from build123d import *
from build123d.topology import SkipClean

# Parameters (mm, degrees)
SKETCH1_R           = 6
BOSS_EXTRUDE1_DEPTH = 5
BOSS_EXTRUDE2_START = -5
BOSS_EXTRUDE2_DEPTH = 5
CUT_EXTRUDE1_START  = -3
SKETCH3_R           = 4.075
CUT_EXTRUDE1_DEPTH  = 3
SKETCH4_W           = 12
SKETCH4_H           = 5
BOSS_EXTRUDE3_DEPTH = 26.5
FILLET1_R           = 6
CUT_EXTRUDE2_DEPTH  = 0.5


with BuildPart() as part:
    # Sketch1 → Boss-Extrude1 (new body)
    with BuildSketch(Plane.XY):
        Circle(SKETCH1_R)
        with BuildLine():
            Line((-2.837252192, 2.925), (2.837252192, 2.925))
            ThreePointArc((2.837252192, 2.925), (0, -4.075), (-2.837252192, 2.925))
        make_face(mode=Mode.SUBTRACT)
    extrude(amount=BOSS_EXTRUDE1_DEPTH)

    # Sketch2 → Boss-Extrude2 (add)
    with BuildSketch(Plane.XY.offset(5).offset(BOSS_EXTRUDE2_START)):
        with BuildLine():
            Line((-6, 0), (-6, 45.2))
            Line((-6, 45.2), (6, 45.2))
            Line((6, 45.2), (6, 0))
            ThreePointArc((6, 0), (0, 6), (-6, 0))
        make_face()
    extrude(amount=BOSS_EXTRUDE2_DEPTH)

    # Sketch3 → Cut-Extrude1 (cut)
    with SkipClean():  # the faces are left unmerged after this step: merging them gives an invalid solid
        with BuildSketch(Plane.XY.offset(5).offset(CUT_EXTRUDE1_START)):
            with Locations(Location((0, 0, 0), (0, 0, 134.127564998))):
                Circle(SKETCH3_R)
        extrude(amount=CUT_EXTRUDE1_DEPTH, mode=Mode.SUBTRACT)

    # Sketch4 → Boss-Extrude3 (add)
    with SkipClean():  # the faces are left unmerged after this step: merging them gives an invalid solid
        with BuildSketch(Plane.XY.offset(5)):
            with Locations((0, 42.7)):
                Rectangle(SKETCH4_W, SKETCH4_H)
        extrude(amount=BOSS_EXTRUDE3_DEPTH)

    # Fillet1
    fillet1_edges = [part.edges().sort_by_distance(p)[0] for p in [
        (-6, 42.7, 31.5),
        (6, 42.7, 31.5),
    ]]
    fillet(fillet1_edges, radius=FILLET1_R - 0.0001)  # a hair under: the kernel refuses the full size

    # Sketch6 → Cut-Extrude2 (cut)
    with BuildSketch(Plane.XY.offset(5)):
        Polygon((-0.872927967, 26.944055952), (-0.872927967, 27.269696978), (0.79598229, 27.269696978), (0.79598229, 26.944055952), (0.10399511, 26.944055952), (0.10399511, 24.094696978), (-0.180940787, 24.094696978), (-0.180940787, 26.944055952), align=None)
    extrude(amount=-CUT_EXTRUDE2_DEPTH, mode=Mode.SUBTRACT)


solid = part.part
The listing builds one solid part. Answer for the finished solid, in the listing's coordinates (mm). Coordinates: 2 decimals unless noted, no trailing zeros. Write each loop counter-clockwise with the first axis right and the second up, starting at its lowest first coordinate (ties: lowest second). Pieces come first, ordered by that corner, then holes. Notation, with made-up numbers: M 42,-20.75 L 59,-20.75 A12 ccw 59,-11.75 Z; hole C 71,11 d6. An arc over 180 degrees is marked long. Use one line per item in the form item = value.
Item 1: Find section D-D, the plane z = 25. Give the vertices of the cut face in (x, y).
Model answer:
outline = M -6,40.2 L 6,40.2 L 6,45.2 L -6,45.2 Z
Item 2: Find section A-A, the plane y = 2. Give the vertices of the cut face in (x, z).
Model answer:
outline = M -6,0 L -3.55,0 L -3.55,5 L -6,5 Z; M 3.55,0 L 6,0 L 6,5 L 3.55,5 Z
Item 3: Given P1, Ø3.5, axis at x = -2, y = 27.5, coming from the +Z side; P2, Ø0.6, axis at x = 0, y = 3.5, coming from the +Z side, each flat-ended and moving along its own axis, determine where each tip first touches the part or whether it passes through.
Model answer:
P1 = 5
P2 = 2
Item 4: Find the intervals of material crossed by probe 1 along X at (y, z) = (0, 2) (3 decimals); probe 2 along Z at (x, y) = (-4.25, 35); probe 3 along Y at (x, z) = (3.5, 13.5), in increasing order.
Model answer:
probe_1 = -6 to -4.075, 4.075 to 6
probe_2 = 0 to 5
probe_3 = 40.2 to 45.2
Item 5: The mould has two halves that part along Y. Classify faces 1 (the face through (0, 23, 5)), 2 (the face through (0, 40.2, 18)), 3 (the face through (0.1, 3.4, 2)), 4 (the face through (0, 2.925, 1)): released by +Y, released by -Y, zero draft, split by the parting line, or undercut.
Model answer:
face_1 = zero draft
face_2 = released by -Y
face_3 = undercut
face_4 = undercut
Item 6: Find section C-C, the plane x = -1.5. Give the vertices of the cut face in (y, z) (1 decimal), plus the area to 3 significant figures.
Model answer:
outline = M -5.8,0 L -3.8,0 L -3.8,5 L -5.8,5 Z; M 2.9,0 L 45.2,0 L 45.2,31.3 L 40.2,31.3 L 40.2,5 L 3.8,5 L 3.8,2 L 2.9,2 Z
area = 350 mm2
Item 7: Find section B-B, the plane z = 3.5. Give the vertices of the cut face in (x, y) (3 decimals).
Model answer:
outline = M -6,0 A6 ccw 6,0 L 6,45.2 L -6,45.2 Z; hole C 0,0 d8.15
